Design review of the part built by this model. Coordinates are the model's own, in mm. A direction names the side the tool comes from. Give positions to 0.01 mm unless a question says otherwise; leave off trailing zeros. Loops run counter-clockwise (first coordinate to the right, second up) from the corner with the lowest first, then second, coordinate; pieces in that order, holes last. Notation, with made-up numbers: (71, 62.25) -> (112, 62.25) arc R23 ccw to (112, 95.25) -> close; hole circle Ø2 at (8, -4). An arc over 180 degrees is marked (long way). Answer in a Markdown table with one row per item. Add a question column.
(1) Consider section B-B on x = -22.5. Write out the cut boundary in (y, z).
(2) For faces 5 (the flat face through (0, 4, 5.299)), 6 (the cylindrical face through (13.95, 8.01, 3.66)), 7 (the flat face through (26, 3, 5)), 8 (the cylindrical face through (-19.327, 1.724, 6.003)), 9 (the cylindrical face through (-28, 2.1, 4.1)), list the 3-axis set-ups (+Z, -Z, +X, -X, +Y, -Y) from which the entire face can be reached by the end or side of a thin tool; tool diameter is ignored.
(3) Draft analysis for pull direction Y (two halves, no side actions). For faces 1 (the cylindrical face through (25.673, 1.724, 6.003)), 2 (the flat face through (0, 9, 5)), 3 (the flat face through (7, 4, 3)), 4 (the flat face through (-26, 3, 5)), state which applies: +Y half, -Y half, draft (parallel to the pull), parting line (faces both ways), or undercut.
(4) Consider section D-D on x = 22. Write out the cut boundary in (y, z), then the cut area to 3 significant figures.
(5) Consider section A-A on y = 6. Write out the cut boundary in (x, z), then the cut area to 3 significant figures.
(6) For pin 1 (2.5 mm diameter, centred on y = 3, z = 5.3, fed in from -X); pin 2 (1.5 mm diameter, centred on x = 6.5, z = 2.5, fed in from -Y); pin 3 (3 mm diameter, centred on x = 22, z = 4.5, fed in from -Y), all flat-tipped, find the tip position at first contact; note any pin that passes through.
(7) Consider section C-C on x = -7. Write out the cut boundary in (y, z), then the cut area to 4 significant figures.
(8) For line 1 (X direction, y = 5.75, z = 8.75); line 2 (X direction, y = 2.25, z = 3); line 3 (X direction, y = 3.5, z = 5.5), list the stretches that pass through material, from the lowest coordinate up.
Autodesk Inventor part; units mm, degrees
sketch "Skizze1" plane through (0, 0, 0) normal (0, 1, 0) x (-1, 0, 0)
  line L0 (30, 0.2989) -> (30, 10.2989)
  line L1 (30, 10.2989) -> (15, 10.2989)
  line L2 (15, 10.2989) -> (15, 5.2989)
  line L3 (15, 5.2989) -> (-15, 5.2989)
  line L4 (-15, 5.2989) -> (-15, 10.2989)
  line L5 (-15, 10.2989) -> (-30, 10.2989)
  line L6 (-30, 10.2989) -> (-30, 0.2989)
  line L7 (-30, 0.2989) -> (30, 0.2989)
  line L8 (0, -2.0598) -> (0, 12.3587)
  point P0 (0, 0)
  dimension "d0" = 30
  dimension "d1" = 5
  dimension "d2" = 15
  dimension "d3" = 15
  dimension "d4" = 15
  dimension "d5" = 5
extrude "Extrusion1" add sketch "Skizze1" along normal blind 9
sketch "Skizze2" plane through (30, 0, 10.2989) normal (1, 0, 0) x (0, 0, -1)
  circle A0 centre (5, 3) radius 1.5
  line L0 (0, 0) -> (0, 9) construction
  line L1 (0, 0) -> (10, 0) construction
  point P0 (10.2989, 0)
  dimension "d8" = 3
  dimension "d9" = 5
  dimension "d43" = 3
  dimension "d60" = 9
  dimension "d61" = 10
extrude "Extrusion2" cut sketch "Skizze2" against normal blind 4
sketch "Skizze4" plane through (-30, 0, 0.2989) normal (-1, 0, 0) x (0, 0, 1)
  circle A0 centre (5, 3) radius 1.5
  circle A1 centre (5, 3) radius 1.5
  line L0 (10, 0) -> (10, 9)
  line L1 (0, 0) -> (10, 0)
  point P0 (-0.2989, 0)
  dimension "d21" = 5
  dimension "d22" = 3
  dimension "d63" = 3
extrude "Extrusion4" cut sketch "Skizze4" against normal blind 4
sketch "Skizze5" plane through (0, 0, 0) normal (0, 1, 0) x (1, 0, 0)
  circle A0 centre (-22.5, -5.2989) radius 1.5
  circle A1 centre (22.5, -5.2989) radius 1.5
  line L0 (-30, -10.2989) -> (-15, -10.2989)
  line L1 (-30, -0.2989) -> (-30, -10.2989)
  line L2 (30, -10.2989) -> (30, -0.2989)
  line L3 (15, -10.2989) -> (30, -10.2989)
  point P0 (0, 0)
  dimension "d25" = 5
  dimension "d26" = 7.5
  dimension "d27" = 7.5
  dimension "d28" = 5
  dimension "d29" = 3
  dimension "d30" = 3
hole "Bohrung1" at (-22.5, 0, 5.2989) at (22.5, 0, 5.2989) direction (0, 1, 0) diameter 3.4 end through all counterbore diameter 6.5 counterbore depth 3.4
sketch "Skizze6" plane through (0, 0, 0) normal (0, -1, 0) x (1, 0, 0)
  circle A0 centre (-7, 2.7989) radius 1.5
  circle A1 centre (7, 2.7989) radius 1.5
  line L0 (-30, 0.2989) -> (-30, 10.2989)
  line L1 (-30, 10.2989) -> (-15, 10.2989)
  line L2 (15, 10.2989) -> (30, 10.2989)
  line L3 (30, 10.2989) -> (30, 0.2989)
  point P0 (0, 0)
  dimension "d33" = 3
  dimension "d34" = 3
  dimension "d36" = 7.5
  dimension "d37" = 7.5
  dimension "d41" = 7
  dimension "d42" = 7
extrude "Extrusion6" cut sketch "Skizze6" against normal blind 4
sketch "Skizze8" plane through (0, 9, 0) normal (0, 1, 0) x (1, 0, 0)
  circle A0 centre (-13.5, -5.2989) radius 1.7
  circle A1 centre (13.5, -5.2989) radius 1.7
  point P0 (0, 0)
extrude "Extrusion8" cut sketch "Skizze8" against normal blind 2
chamfer "Fase1" distance 0.5 angle 45 4 edges at (-30, 4.5, 0.2989) (0, 0, 0.2989) (0, 9, 0.2989) (30, 4.5, 0.2989)
equation "\"d2\" = 0.5 * d0"
equation "\"d9\" = 0.5 * d61"
equation "\"d33\" = d34"
properties part number "Fuehrungslagerhalter_v2" material "PBT-Kunststoff"
Values follow:
| question | item | result |
|---|---|---|
| 1 | outline | (0, 0.8) -> (0.5, 0.3) -> (8.5, 0.3) -> (9, 0.8) -> (9, 3.6) -> (3.4, 3.6) -> (3.4, 2.05) -> (0, 2.05) -> close; (0, 8.55) -> (3.4, 8.55) -> (3.4, 7) -> (9, 7) -> (9, 10.3) -> (0, 10.3) -> close |
| 2 | face 5 | +Z, +Y, -Y |
| 2 | face 6 | +Y |
| 2 | face 7 | +X |
| 2 | face 8 | -Y |
| 2 | face 9 | -X |
| 3 | face 1 | draft |
| 3 | face 2 | +Y half |
| 3 | face 3 | -Y half |
| 3 | face 4 | undercut |
| 4 | outline | (0, 0.8) -> (0.5, 0.3) -> (8.5, 0.3) -> (9, 0.8) -> (9, 3.67) -> (3.4, 3.67) -> (3.4, 2.09) -> (0, 2.09) -> close; (0, 8.51) -> (3.4, 8.51) -> (3.4, 6.92) -> (9, 6.92) -> (9, 10.3) -> (0, 10.3) -> close |
| 4 | area | 49.7 mm2 |
| 5 | outline | (-30, 0.8) -> (-29.5, 0.3) -> (29.5, 0.3) -> (30, 0.8) -> (30, 10.3) -> (15, 10.3) -> (15, 5.3) -> (-15, 5.3) -> (-15, 10.3) -> (-30, 10.3) -> close; hole circle Ø3.4 at (-22.5, 5.3); hole circle Ø3.4 at (22.5, 5.3) |
| 5 | area | 432 mm2 |
| 6 | pin 1 | x = -26 |
| 6 | pin 2 | y = 4 |
| 6 | pin 3 | y = 3.4 |
| 7 | outline | (0, 0.8) -> (0.5, 0.3) -> (8.5, 0.3) -> (9, 0.8) -> (9, 5.3) -> (0, 5.3) -> (0, 4.3) -> (4, 4.3) -> (4, 1.3) -> (0, 1.3) -> close |
| 7 | area | 32.75 mm2 |
| 8 | line 1 | -30 to -15, 15 to 30 |
| 8 | line 2 | -30 to -24.8, -20.2 to -8.49, -5.51 to 5.51, 8.49 to 20.2, 24.8 to 30 |
| 8 | line 3 | -26 to -24.19, -20.81 to -15, 15 to 20.81, 24.19 to 26 |
